```python
from build123d import *
from build123d.topology import SkipClean

# Parameters (mm, degrees)
ESQUISSE1_W                  = 50
ESQUISSE1_H                  = 20
BOSS_EXTRU_1_DEPTH           = 9
ESQUISSE2_W                  = 30
ESQUISSE2_H                  = 30
BOSS_EXTRU_2_DEPTH           = 9
ENL_V_MAT_EXTRU_1_DEPTH      = 85.297093663
ENL_V_MAT_EXTRU_1_DEPTH_BACK = 85.297093663
ESQUISSE3_R                  = 8.75
ESQUISSE3_R_2                = 1.65
ENL_V_MAT_EXTRU_2_DEPTH      = 85.297093663
ENL_V_MAT_EXTRU_2_DEPTH_BACK = 85.297093663
ESQUISSE4_R                  = 4
CONG_1_R                     = 10
ESQUISSE6_R                  = 19
ESQUISSE6_R_2                = 14
BOSS_EXTRU_3_DEPTH           = 9
ENL_V_MAT_EXTRU_4_DEPTH      = 90.319650693


with BuildPart() as part:
    # Esquisse1 → Boss.-Extru.1 (new body)
    with BuildSketch(Plane.XY):
        with Locations((25, 10)):
            Rectangle(ESQUISSE1_W, ESQUISSE1_H)
    extrude(amount=BOSS_EXTRU_1_DEPTH)

    # Esquisse2 → Boss.-Extru.2 (add)
    with BuildSketch(Plane.XY.offset(9)):
        with Locations((65, 10)):
            Rectangle(ESQUISSE2_W, ESQUISSE2_H)
    extrude(amount=-BOSS_EXTRU_2_DEPTH)

    # Esquisse3 → Enlèv. mat.-Extru.1 (cut, two sides: drawn at the far end of the back side and taken through both)
    with BuildSketch(Plane.XY.offset(9).offset(-ENL_V_MAT_EXTRU_1_DEPTH_BACK)):
        with Locations((65, 10)):
            Circle(ESQUISSE3_R)
        with Locations((65, -1)):
            Circle(ESQUISSE3_R_2)
        with Locations((55.473720558, 4.5)):
            Circle(ESQUISSE3_R_2)
        with Locations((55.473720558, 15.5)):
            Circle(ESQUISSE3_R_2)
        with Locations((65, 21)):
            Circle(ESQUISSE3_R_2)
        with Locations((74.526279442, 15.5)):
            Circle(ESQUISSE3_R_2)
        with Locations((74.526279442, 4.5)):
            Circle(ESQUISSE3_R_2)
    extrude(amount=ENL_V_MAT_EXTRU_1_DEPTH + ENL_V_MAT_EXTRU_1_DEPTH_BACK, mode=Mode.SUBTRACT)

    # Esquisse4 → Enlèv. mat.-Extru.2 (cut, two sides: drawn at the far end of the back side and taken through both)
    with BuildSketch(Plane.XY.offset(9).offset(-ENL_V_MAT_EXTRU_2_DEPTH_BACK)):
        with Locations((10, 10)):
            Circle(ESQUISSE4_R)
    extrude(amount=ENL_V_MAT_EXTRU_2_DEPTH + ENL_V_MAT_EXTRU_2_DEPTH_BACK, mode=Mode.SUBTRACT)

    # Congé1
    cong_1_edges = [part.edges().sort_by_distance(p)[0] for p in [
        (0, 0, 4.5),
        (0, 20, 4.5),
    ]]
    fillet(cong_1_edges, radius=CONG_1_R - 0.0001)  # a hair under: the kernel refuses the full size

    # Esquisse6 → Boss.-Extru.3 (add)
    with BuildSketch(Plane.XY.offset(9)):
        with Locations((65, 10)):
            Circle(ESQUISSE6_R)
        with Locations((65, 10)):
            Circle(ESQUISSE6_R_2, mode=Mode.SUBTRACT)
    extrude(amount=-BOSS_EXTRU_3_DEPTH)

    # Esquisse7 → Enlèv. mat.-Extru.4 (cut, through all)
    with SkipClean():  # the faces are left unmerged after this step: merging them gives an invalid solid
        with BuildSketch(Plane.XY.offset(9)):
            with BuildLine():
                Line((48.844505579, 0), (48.844505579, -10.5))
                Line((48.844505579, -10.5), (84.844505579, -10.5))
                Line((84.844505579, -10.5), (84.844505579, 30.5))
                Line((84.844505579, 30.5), (48.844505579, 30.5))
                Line((48.844505579, 30.5), (48.844505579, 20))
                ThreePointArc((48.844505579, 20), (84, 10), (48.844505579, 0))
            make_face()
        extrude(amount=-ENL_V_MAT_EXTRU_4_DEPTH, mode=Mode.SUBTRACT)


solid = part.part
```
Read the model definition and answer for the solid it produces. Units are mm, in the model's axes. A direction names the side the tool comes from. Give positions to 0.01 mm unless a question says otherwise; leave off trailing zeros. Order: outer loops, then holes, each group sorted by start corner. A loop starts at its lowest first (then second) coordinate and runs counter-clockwise, first axis right, second up.
(1) For a pull along X with two mould halves and no side action, classify faces 4 (the cylindrical face through (76.05, 14.87, 4.44)), 5 (the flat face through (51, 10, 0)), 6 (the cylindrical face through (3.01, 2.85, 4.56)) as released by +X, released by -X, zero draft, split by the parting line, or undercut.
(2) Given pin 1 (2 mm diameter, centred on x = 67, z = 3.5, fed in from -Y); pin 2 (4.5 mm diameter, centred on x = 37, z = 5, fed in from +Y); pin 3 (2 mm diameter, centred on y = 21.5, z = 1.5, fed in from -X), each flat-ended and moving along its own axis, determine where each tip first touches the part or whether it passes through.
(3) For faces 1 (the cylindrical face through (57, 14.87, 4.44)), 2 (the flat face through (29, 20, 4)), 3 (the flat face through (29, 0, 4)), determine the directions among +Z, -Z, +X, -X, +Y, -Y from which every point of the face is accessible in a straight line to the end or side of a thin tool.
(4) Find section A-A (z = 2). Give the number of separate pieces and of enclosed holes in the cut face, plus the area to 3 significant figures.
(5) Straight lines are drawn through the part: L1, parallel to X at y = 10, z = 7; L2, parallel to Y at x = 65, z = 7.25; L3, parallel to Y at x = 74, z = 6.25. For each, find the intervals that lie inside material, in ascending order.
(6) Find section B-B (x = 65). Give the vertices of the cut face in (y, z).
(7) Find section D-D (x = 12.5). Give the vertices of the cut face in (y, z).
(8) Find section C-C (y = 4.5). Give the vertices of the cut face in (x, z).
Result sheet:
1. face 4: undercut
1. face 5: zero draft
1. face 6: released by -X
2. pin 1: stops at y = -8.97
2. pin 2: stops at y = 20
2. pin 3: stops at x = 49.16
3. face 1: +Z, -Z
3. face 2: +Z, -Z, -X, +Y
3. face 3: +Z, -Z, -X, -Y
4. separate pieces: 1
4. enclosed holes: 8
4. area: 1,690 mm2
5. L1: x = 0 to 6, 14 to 56.25, 73.75 to 84
5. L2: y = -9 to -2.65, 0.65 to 1.25, 18.75 to 19.35, 22.65 to 29
5. L3: y = -6.73 to 2.94, 6.06 to 13.94, 17.06 to 26.73
6. outline: (-9, 0) - (-2.65, 0) - (-2.65, 9) - (-9, 9) - close; (0.65, 0) - (1.25, 0) - (1.25, 9) - (0.65, 9) - close; (18.75, 0) - (19.35, 0) - (19.35, 9) - (18.75, 9) - close; (22.65, 0) - (29, 0) - (29, 9) - (22.65, 9) - close
7. outline: (0, 0) - (6.88, 0) - (6.88, 9) - (0, 9) - close; (13.12, 0) - (20, 0) - (20, 9) - (13.12, 9) - close
8. outline: (1.65, 0) - (53.82, 0) - (53.82, 9) - (1.65, 9) - close; (57.12, 0) - (58.19, 0) - (58.19, 9) - (57.12, 9) - close; (71.81, 0) - (72.88, 0) - (72.88, 9) - (71.81, 9) - close; (76.18, 0) - (83.19, 0) - (83.19, 9) - (76.18, 9) - close
